```python
from build123d import *

# Parameters (mm, degrees)
CUT_EXTRUDE1_DEPTH = 23.549944568


with BuildPart() as part:
    # Sketch1 → Revolve1 (revolve)
    with BuildSketch(Plane(origin=(0, 0, 0), x_dir=(1, 0, 0), z_dir=(0, 1, 0)), mode=Mode.PRIVATE) as revolve1_sk:
        Polygon((-4, 0), (-8, 0), (-8, 3), (-11.5, 3), (-13.5, 3.75), (-13.5, 5.25), (-11.5, 6), (-8, 6), (-8, 15), (-4, 15), align=None)
    revolve(revolve1_sk.sketch.rotate(Axis((0, 0, 0), (0, 0, -1)), 180), axis=Axis((0, 0, 0), (0, 0, -1)))

    # Sketch2 → Cut-Extrude1 (cut, through all)
    with BuildSketch(Plane.XY.offset(-3)):
        with BuildLine():
            Line((-2.5, 13.266499161), (-1.354141447, 11.281813929))
            ThreePointArc((-1.354141447, 11.281813929), (0, 10.5), (1.354141447, 11.281813929))
            Line((1.354141447, 11.281813929), (2.5, 13.266499161))
            ThreePointArc((2.5, 13.266499161), (0, 13.5), (-2.5, 13.266499161))
        make_face()
        with BuildLine():
            Line((4.468186071, 12.739125293), (4.468186071, 10.447408186))
            ThreePointArc((4.468186071, 10.447408186), (5.25, 9.09326674), (6.813627858, 9.09326674))
            Line((6.813627858, 9.09326674), (8.79831309, 10.239125293))
            ThreePointArc((8.79831309, 10.239125293), (6.75, 11.691342951), (4.468186071, 12.739125293))
        make_face()
        with BuildLine():
            Line((10.239125293, 8.79831309), (9.09326674, 6.813627858))
            ThreePointArc((9.09326674, 6.813627858), (9.09326674, 5.25), (10.447408186, 4.468186071))
            Line((10.447408186, 4.468186071), (12.739125293, 4.468186071))
            ThreePointArc((12.739125293, 4.468186071), (11.691342951, 6.75), (10.239125293, 8.79831309))
        make_face()
        with BuildLine():
            Line((13.266499161, 2.5), (11.281813929, 1.354141447))
            ThreePointArc((11.281813929, 1.354141447), (10.5, 0), (11.281813929, -1.354141447))
            Line((11.281813929, -1.354141447), (13.266499161, -2.5))
            ThreePointArc((13.266499161, -2.5), (13.5, 0), (13.266499161, 2.5))
        make_face()
        with BuildLine():
            Line((12.739125293, -4.468186071), (10.447408186, -4.468186071))
            ThreePointArc((10.447408186, -4.468186071), (9.09326674, -5.25), (9.09326674, -6.813627858))
            Line((9.09326674, -6.813627858), (10.239125293, -8.79831309))
            ThreePointArc((10.239125293, -8.79831309), (11.691342951, -6.75), (12.739125293, -4.468186071))
        make_face()
        with BuildLine():
            Line((8.79831309, -10.239125293), (6.813627858, -9.09326674))
            ThreePointArc((6.813627858, -9.09326674), (5.25, -9.09326674), (4.468186071, -10.447408186))
            Line((4.468186071, -10.447408186), (4.468186071, -12.739125293))
            ThreePointArc((4.468186071, -12.739125293), (6.75, -11.691342951), (8.79831309, -10.239125293))
        make_face()
        with BuildLine():
            Line((2.5, -13.266499161), (1.354141447, -11.281813929))
            ThreePointArc((1.354141447, -11.281813929), (0, -10.5), (-1.354141447, -11.281813929))
            Line((-1.354141447, -11.281813929), (-2.5, -13.266499161))
            ThreePointArc((-2.5, -13.266499161), (0, -13.5), (2.5, -13.266499161))
        make_face()
        with BuildLine():
            Line((-4.468186071, -12.739125293), (-4.468186071, -10.447408186))
            ThreePointArc((-4.468186071, -10.447408186), (-5.25, -9.09326674), (-6.813627858, -9.09326674))
            Line((-6.813627858, -9.09326674), (-8.79831309, -10.239125293))
            ThreePointArc((-8.79831309, -10.239125293), (-6.75, -11.691342951), (-4.468186071, -12.739125293))
        make_face()
        with BuildLine():
            Line((-10.239125293, -8.79831309), (-9.09326674, -6.813627858))
            ThreePointArc((-9.09326674, -6.813627858), (-9.09326674, -5.25), (-10.447408186, -4.468186071))
            Line((-10.447408186, -4.468186071), (-12.739125293, -4.468186071))
            ThreePointArc((-12.739125293, -4.468186071), (-11.691342951, -6.75), (-10.239125293, -8.79831309))
        make_face()
        with BuildLine():
            Line((-13.266499161, -2.5), (-11.281813929, -1.354141447))
            ThreePointArc((-11.281813929, -1.354141447), (-10.5, 0), (-11.281813929, 1.354141447))
            Line((-11.281813929, 1.354141447), (-13.266499161, 2.5))
            ThreePointArc((-13.266499161, 2.5), (-13.5, 0), (-13.266499161, -2.5))
        make_face()
        with BuildLine():
            Line((-12.739125293, 4.468186071), (-10.447408186, 4.468186071))
            ThreePointArc((-10.447408186, 4.468186071), (-9.09326674, 5.25), (-9.09326674, 6.813627858))
            Line((-9.09326674, 6.813627858), (-10.239125293, 8.79831309))
            ThreePointArc((-10.239125293, 8.79831309), (-11.691342951, 6.75), (-12.739125293, 4.468186071))
        make_face()
        with BuildLine():
            Line((-8.79831309, 10.239125293), (-6.813627858, 9.09326674))
            ThreePointArc((-6.813627858, 9.09326674), (-5.25, 9.09326674), (-4.468186071, 10.447408186))
            Line((-4.468186071, 10.447408186), (-4.468186071, 12.739125293))
            ThreePointArc((-4.468186071, 12.739125293), (-6.75, 11.691342951), (-8.79831309, 10.239125293))
        make_face()
    extrude(amount=-CUT_EXTRUDE1_DEPTH, mode=Mode.SUBTRACT)


solid = part.part
```
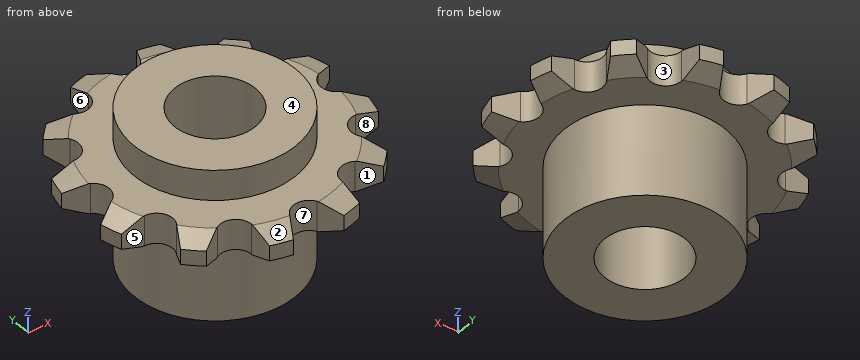
Work out the finished part from the listing and answer in its coordinate system (mm). Face numbers are marked on the shaded views. A direction names the side the tool comes from. Round coordinates to 2 decimals unless told otherwise and drop trailing zeros. Order: outer loops, then holes, each group sorted by start corner. A loop starts at its lowest first (then second) coordinate and runs counter-clockwise, first axis right, second up.
Q1. A cutting plane is placed at D-D, the plane x = 6.25. Determine the outline of the cut face in (y, z).
Solution:
outline: (-8.9, -6) - (-4.99, -6) - (-4.99, -15) - (4.99, -15) - (4.99, -6) - (8.9, -6) - (8.9, -3) - (4.99, -3) - (4.99, 0) - (-4.99, 0) - (-4.99, -3) - (-8.9, -3) - close
Q2. A tool of negligible diameter and unlimited length cuts with its end or side. For the marked faces 5, 6, 7 and 8, from which of +Z, -Z, +X, -X, +Y, -Y can it reach the whole face along a straight path? Write none if from no direction.
Solution:
face 5: +Z, -Z, -X, -Y
face 6: +Z, -Z, -X, +Y
face 7: +Z, -Z, -Y
face 8: +Z, -Z, +X, -Y
Q3. Given pin 1 Ø0.7 at (x, z) = (-11.5, -4.5) entering from -Y; pin 2 Ø1.8 at (y, z) = (-11, -4.5) entering from +X; pin 3 Ø6 at (y, z) = (8, -8) entering from -X; pin 4 Ø7 at (x, y) = (0, 0) entering from +Z, each flat-ended and moving along its own axis, determine where each tip first touches the part or whether it passes through.
Solution:
pin 1: stops at y = -4.47
pin 2: stops at x = 8.96
pin 3: stops at x = -10.24
pin 4: passes through
Q4. Find the intervals of material crossed by line 1 along Y through (x, z) = (0, -11); line 2 along Y through (x, z) = (-1.5, -12); line 3 along Z through (x, y) = (-8.5, 1.25), in increasing order.
Solution:
line 1: y = -8 to -4, 4 to 8
line 2: y = -7.86 to -3.71, 3.71 to 7.86
line 3: z = -6 to -3
Q5. A cutting plane is placed at C-C, the plane z = -11.25. Determine the outline of the cut face in (x, y).
Solution:
outline: circle Ø16 at (0, 0); hole circle Ø8 at (0, 0)
Q6. The mould has two halves that part along X. Classify the marked faces 1, 2, 3 and 4: pulls with the +X half, pulls with the -X half, needs draft (parallel to the pull), parting line crosses it, or undercut.
Solution:
face 1: undercut
face 2: pulls with the -X half
face 3: undercut
face 4: needs draft
Q7. A cutting plane is placed at A-A, the plane x = 0. Determine the outline of the cut face in (y, z).
Solution:
outline: (-10.5, -6) - (-8, -6) - (-8, -15) - (-4, -15) - (-4, 0) - (-8, 0) - (-8, -3) - (-10.5, -3) - close; (4, -15) - (8, -15) - (8, -6) - (10.5, -6) - (10.5, -3) - (8, -3) - (8, 0) - (4, 0) - close
